Source: three-view drawing plus pictorial views. Frame: mm from the lowest corner of the part. A direction names the side the tool comes from. Give positions to 0.01 mm unless a question says otherwise; leave off trailing zeros. Loops run counter-clockwise (first coordinate to the right, second up) from the corner with the lowest first, then second, coordinate; pieces in that order, holes last.
1. Section D-D, the plane z = 24. Output: boundary loops of the cut face in (x, y), then the cut area to 3 significant figures.
2. Draft query along Z for the marked faces 1, 2 and 3. Return one class per face: +Z half, -Z half, draft (parallel to the pull), parting line (faces both ways), or undercut.
3. Material intervals for line 1 along Y through (x, z) = (36, 103.75); line 2 along Z through (x, y) = (14, 62); line 3 along X through (y, z) = (46, 1), sorted ascending.
4. Section C-C, the plane y = 46. Output: boundary loops of the cut face in (x, z), then the cut area to 3 significant figures.
5. Section B-B, the plane x = 36. Output: boundary loops of the cut face in (y, z).
6. Section A-A, the plane y = 71. Output: boundary loops of the cut face in (x, z).
7. Access query for the marked faces 4 and 5. Directions: +Z, -Z, +X, -X, +Y, -Y. A direction counts if a zero-diameter tool reaches every point of the face in a straight line with its end or side. Return the directions, or none.
8. First-contact query: P1, Ø1.5, axis at y = 11, z = 58.5, coming from the +X side; P2, Ø2.5, axis at y = 71, z = 52.5, coming from the -X side; P3, Ø2, axis at x = 33.5, z = 84, coming from the +Y side; P4, Ø6.5, axis at x = 17, y = 70.5, coming from the +Z side. Flat tips, straight axial feed; report the tip coordinate or a pass-through.
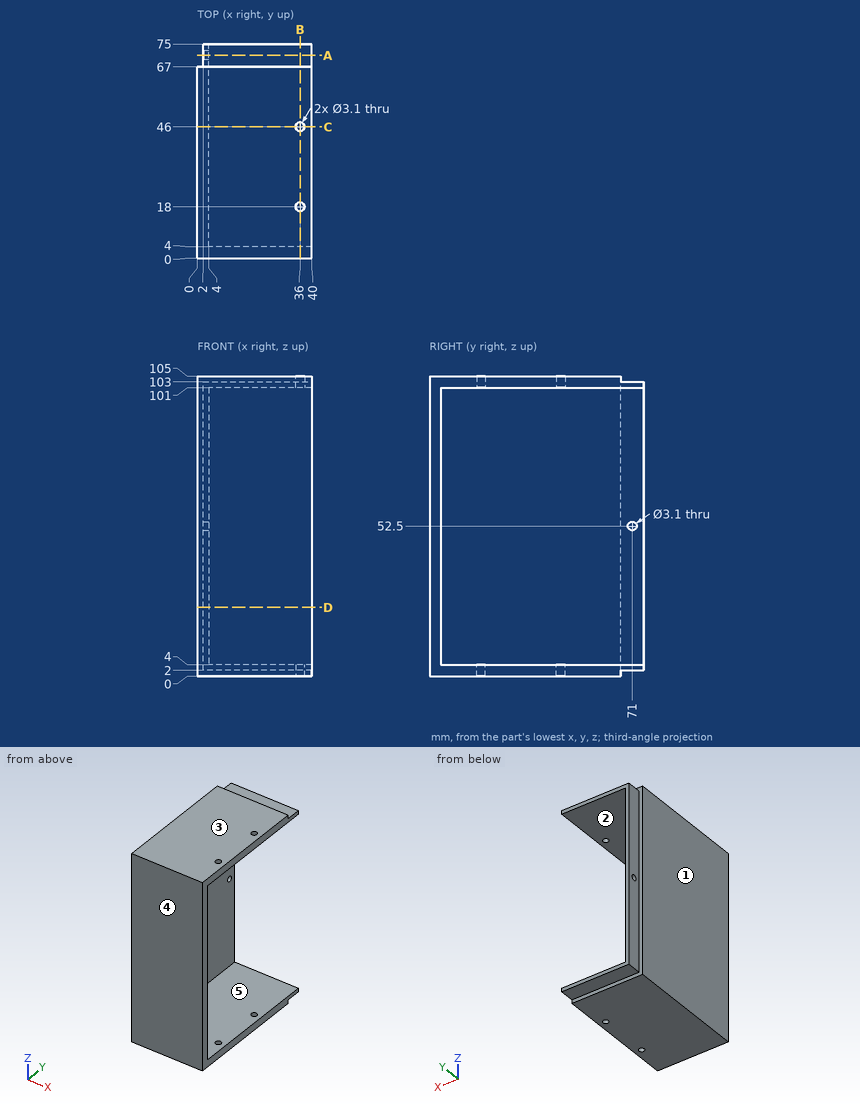
Answers below:
1. outline: (0, 0) - (40, 0) - (40, 4) - (4, 4) - (4, 75) - (2, 75) - (2, 67) - (0, 67) - close
1. area: 428 mm2
2. face 1: draft
2. face 2: undercut
2. face 3: +Z half
3. line 1: y = 0 to 16.45, 19.55 to 44.45, 47.55 to 67
3. line 2: z = 0 to 4, 101 to 105
3. line 3: x = 0 to 34.45, 37.55 to 40
4. outline: (0, 0) - (34.45, 0) - (34.45, 4) - (4, 4) - (4, 101) - (34.45, 101) - (34.45, 105) - (0, 105) - close; (37.55, 0) - (40, 0) - (40, 4) - (37.55, 4) - close; (37.55, 101) - (40, 101) - (40, 105) - (37.55, 105) - close
4. area: 683 mm2
5. outline: (0, 0) - (16.45, 0) - (16.45, 4) - (4, 4) - (4, 101) - (16.45, 101) - (16.45, 105) - (0, 105) - close; (19.55, 0) - (44.45, 0) - (44.45, 4) - (19.55, 4) - close; (19.55, 101) - (44.45, 101) - (44.45, 105) - (19.55, 105) - close; (47.55, 0) - (67, 0) - (67, 2) - (75, 2) - (75, 4) - (47.55, 4) - close; (47.55, 101) - (75, 101) - (75, 103) - (67, 103) - (67, 105) - (47.55, 105) - close
6. outline: (2, 2) - (40, 2) - (40, 4) - (4, 4) - (4, 50.95) - (2, 50.95) - close; (2, 54.05) - (4, 54.05) - (4, 101) - (40, 101) - (40, 103) - (2, 103) - close
7. face 4: +Z, -Z, +X, -X, -Y
7. face 5: +X, +Y
8. P1: stops at x = 4
8. P2: passes through
8. P3: stops at y = 4
8. P4: stops at z = 103
